Could you check a few things on this model? Use its own coordinates, in mm. Round coordinates to 2 decimals unless told otherwise and drop trailing zeros. Loops run counter-clockwise (first coordinate to the right, second up) from the corner with the lowest first, then second, coordinate; pieces in that order, holes last. Notation, with made-up numbers: (22.5, -17.75) -> (71.5, -17.75) arc R31 cw to (71.5, 19.25) -> close; hole circle Ø3 at (-5.75, 28.25). An arc over 180 degrees is marked (long way). Write each question's results on one line, items separated by ' | '.
from build123d import *

# Parameters (mm, degrees)
SKETCH1_W           = 19.05
SKETCH1_H           = 19.05
BOSS_EXTRUDE1_DEPTH = 1828.8
SKETCH2_W           = 12.7
SKETCH2_H           = 12.7
CUT_EXTRUDE1_DEPTH  = 1829.8
SKETCH3_R           = 3.175
CUT_EXTRUDE2_DEPTH  = 20.05


with BuildPart() as part:
    # Sketch1 → Boss-Extrude1 (new body)
    with BuildSketch(Plane(origin=(0, 0, 0), x_dir=(1, 0, 0), z_dir=(0, 1, 0))):
        with Locations((9.525, 9.525)):
            Rectangle(SKETCH1_W, SKETCH1_H)
    extrude(amount=BOSS_EXTRUDE1_DEPTH)

    # Sketch2 → Cut-Extrude1 (cut, through all)
    with BuildSketch(Plane(origin=(0, 1828.8, 0), x_dir=(1, 0, 0), z_dir=(0, 1, 0))):
        with Locations((9.525, 9.525)):
            Rectangle(SKETCH2_W, SKETCH2_H)
    extrude(amount=-CUT_EXTRUDE1_DEPTH, mode=Mode.SUBTRACT)

    # Sketch3 → Cut-Extrude2 (cut, through all)
    with BuildSketch(Plane.XY):
        with Locations((9.525, 1727.2)):
            Circle(SKETCH3_R)
        with Locations((9.525, 1524)):
            Circle(SKETCH3_R)
        with Locations((9.525, 1219.2)):
            Circle(SKETCH3_R)
        with Locations((9.525, 914.4)):
            Circle(SKETCH3_R)
        with Locations((9.525, 406.4)):
            Circle(SKETCH3_R)
        with Locations((9.525, 609.6)):
            Circle(SKETCH3_R)
    extrude(amount=-CUT_EXTRUDE2_DEPTH, mode=Mode.SUBTRACT)


solid = part.part
1) I'm going to push a flat-ended pin straight in: pin 1 (5 mm diameter, centred on x = 9.525, y = 1524, fed in from +Z). Where does the tip first touch, or does it pass through?
Model answer:
pin 1: passes through
2) I need wall thicknesses on line 1 (Z direction, x = 6.5, y = 864.5) (3 decimals); line 2 (X direction, y = 451, z = -9.5) (3 decimals); line 3 (X direction, y = 1219.2, z = -1.3). Which ranges of each line are inside material? Lowest first, please.
Model answer:
line 1: z = -19.05 to -15.875, -3.175 to 0 | line 2: x = 0 to 3.175, 15.875 to 19.05 | line 3: x = 0 to 6.35, 12.7 to 19.05
3) I want a section at B-B, the plane y = 1696. Write out the boundary of the cut face in (x, z) (3 decimals).
Model answer:
outline: (0, -19.05) -> (19.05, -19.05) -> (19.05, 0) -> (0, 0) -> close; hole (3.175, -15.875) -> (15.875, -15.875) -> (15.875, -3.175) -> (3.175, -3.175) -> close
4) I want a section at A-A, the plane z = -11. Write out the boundary of the cut face in (x, y) (3 decimals).
Model answer:
outline: (0, 0) -> (3.175, 0) -> (3.175, 1828.8) -> (0, 1828.8) -> close; (15.875, 0) -> (19.05, 0) -> (19.05, 1828.8) -> (15.875, 1828.8) -> close
